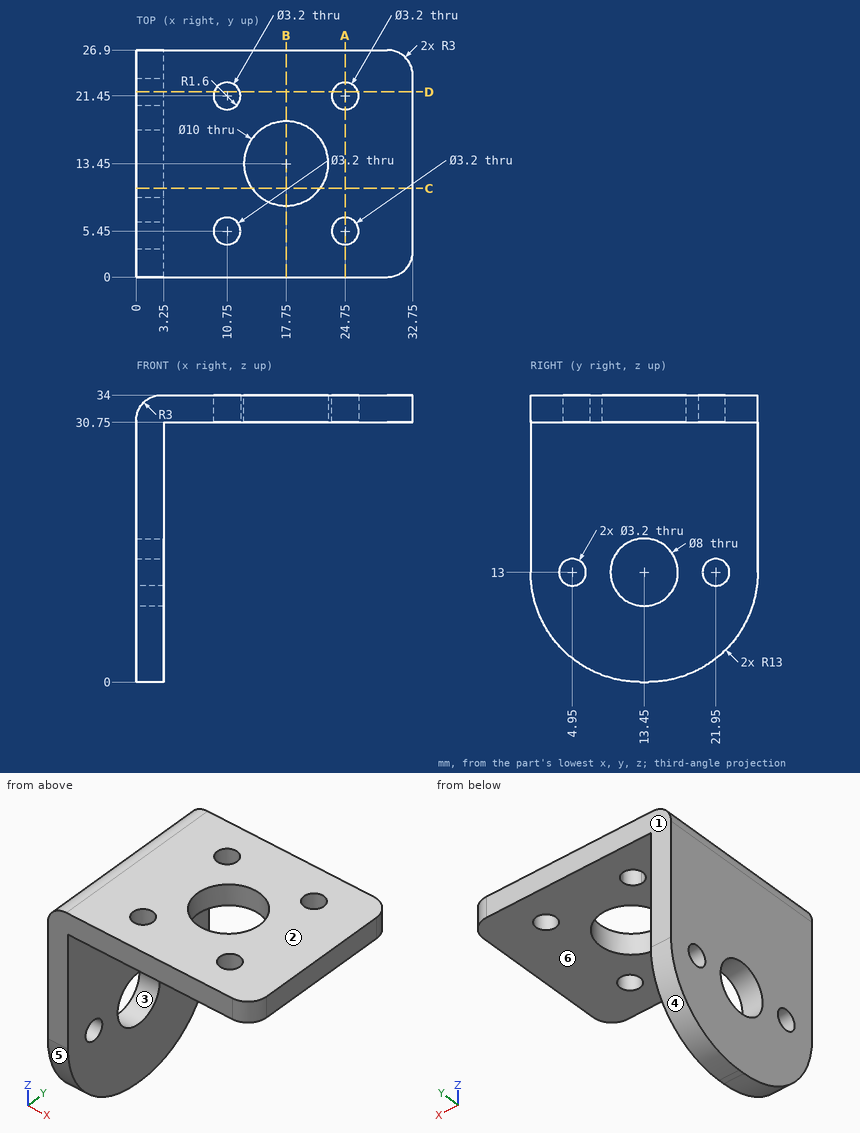
Job drawing, mm, ordinate dimensions from the low corner. One solid piece. A direction names the side the tool comes from. Round coordinates to 2 decimals unless told otherwise and drop trailing zeros. Write each loop counter-clockwise with the first axis right and the second up, starting at its lowest first coordinate (ties: lowest second). Pieces come first, ordered by that corner, then holes. Notation, with made-up numbers: (57.25, 11) -> (115.25, 11) arc R28 ccw to (115.25, 31) -> close; hole circle Ø9 at (85, 61.25). An arc over 180 degrees is marked (long way). Answer as a JSON object with one key per item and string values.
(1) Band-saw the part on D-D, the plane y = 21.95. List the corners of the cut face in (x, z), then the cut area to 3 significant figures.
Reported:
{"outline": "(0, 2.79) -> (3.25, 2.79) -> (3.25, 11.4) -> (0, 11.4) -> close; (0, 14.6) -> (3.25, 14.6) -> (3.25, 30.75) -> (9.23, 30.75) -> (9.23, 34) -> (3, 34) arc R3 ccw to (0, 31) -> close; (12.27, 30.75) -> (23.23, 30.75) -> (23.23, 34) -> (12.27, 34) -> close; (26.27, 30.75) -> (32.75, 30.75) -> (32.75, 34) -> (26.27, 34) -> close", "area": "165 mm^2"}
(2) Probe probe 1 along Y at (x, z) = (2.25, 13); probe 2 along Y at (x, z) = (10.75, 32.05); probe 3 along Y at (x, z) = (17.75, 32.3). List the from-to ranges inside material, lowest first. Write a range as [from, to].
Reported:
{"probe 1": "y = [0, 3.35], [6.55, 9.45], [17.45, 20.35], [23.55, 26.9]", "probe 2": "y = [0, 3.85], [7.05, 19.85], [23.05, 26.9]", "probe 3": "y = [0, 8.45], [18.45, 26.9]"}
(3) Pin check, flat tips, straight feed: P1, Ø5, axis at x = 24.75, y = 21.45, coming from the -Z side; P2, Ø13, axis at y = 13.45, z = 13, coming from the +X side. Stop position of each tip, or through.
Reported:
{"P1": "stops at z = 30.75", "P2": "stops at x = 3.25"}
(4) Which spindle directions (+Z, -Z, +X, -X, +Y, -Y) get a long thin tool onto all of the face, cutting with end or side? Do the marked faces 5 and 6. Say none if no direction does.
Reported:
{"face 5": "-Z, +X, -X, -Y", "face 6": "-Z, +X, +Y, -Y"}
(5) Band-saw the part on A-A, the plane x = 24.75. List the corners of the cut face in (y, z), then the cut area to 3 significant figures.
Reported:
{"outline": "(0, 30.75) -> (3.85, 30.75) -> (3.85, 34) -> (0, 34) -> close; (7.05, 30.75) -> (19.85, 30.75) -> (19.85, 34) -> (7.05, 34) -> close; (23.05, 30.75) -> (26.9, 30.75) -> (26.9, 34) -> (23.05, 34) -> close", "area": "66.6 mm^2"}
(6) Two-plate mould, pull along Z, no slides. Class the marked faces 1, 2, 3 and 4: +Z half, -Z half, draft (parallel to the pull), parting line (faces both ways), or undercut.
Reported:
{"face 1": "draft", "face 2": "+Z half", "face 3": "undercut", "face 4": "-Z half"}
(7) Band-saw the part on B-B, the plane x = 17.75. List the corners of the cut face in (y, z), then the cut area to 3 significant figures.
Reported:
{"outline": "(0, 30.75) -> (8.45, 30.75) -> (8.45, 34) -> (0, 34) -> close; (18.45, 30.75) -> (26.9, 30.75) -> (26.9, 34) -> (18.45, 34) -> close", "area": "54.9 mm^2"}
(8) Band-saw the part on C-C, the plane y = 10.5. List the corners of the cut face in (x, z), then the cut area to 3 significant figures.
Reported:
{"outline": "(0, 0.24) -> (3.25, 0.24) -> (3.25, 10.3) -> (0, 10.3) -> close; (0, 15.7) -> (3.25, 15.7) -> (3.25, 30.75) -> (13.71, 30.75) -> (13.71, 34) -> (3, 34) arc R3 ccw to (0, 31) -> close; (21.79, 30.75) -> (32.75, 30.75) -> (32.75, 34) -> (21.79, 34) -> close", "area": "160 mm^2"}
